from build123d import *

# Parameters (mm, degrees)
SKETCH1_R           = 7.5
BOSS_EXTRUDE2_DEPTH = 2.5
SKETCH1_6_R         = 2.5
CUT_EXTRUDE1_DEPTH  = 3.5
SKETCH1_7_R         = 3.5
SKETCH1_7_R_2       = 2.5
BOSS_EXTRUDE3_DEPTH = 4


with BuildPart() as part:
    # Sketch1 → Boss-Extrude2 (new body)
    with BuildSketch(Plane(origin=(0, 0, 0), x_dir=(1, 0, 0), z_dir=(0, 1, 0))):
        Circle(SKETCH1_R)
    extrude(amount=BOSS_EXTRUDE2_DEPTH)

    # Sketch1<6> → Cut-Extrude1 (cut)
    with BuildSketch(Plane(origin=(0, 0, 0), x_dir=(1, 0, 0), z_dir=(0, 1, 0))):
        Circle(SKETCH1_6_R)
    extrude(amount=CUT_EXTRUDE1_DEPTH, mode=Mode.SUBTRACT)

    # Sketch1<7> → Boss-Extrude3 (add)
    with BuildSketch(Plane(origin=(0, 0, 0), x_dir=(1, 0, 0), z_dir=(0, 1, 0))):
        Circle(SKETCH1_7_R)
        Circle(SKETCH1_7_R_2, mode=Mode.SUBTRACT)
    extrude(amount=BOSS_EXTRUDE3_DEPTH)


solid = part.part
Input: part model. Units: mm. Frame: model coordinates. A direction names the side the tool comes from. Round coordinates to 2 decimals unless told otherwise and drop trailing zeros. Order: outer loops, then holes, each group sorted by start corner. A loop starts at its lowest first (then second) coordinate and runs counter-clockwise, first axis right, second up.
1. Cut plane B-B, the plane z = 2.25. Output: boundary loops of the cut face in (x, y), then the cut area to 3 significant figures.
The answers:
outline: (-7.15, 0) - (-1.09, 0) - (-1.09, 4) - (-2.68, 4) - (-2.68, 2.5) - (-7.15, 2.5) - close; (1.09, 0) - (7.15, 0) - (7.15, 2.5) - (2.68, 2.5) - (2.68, 4) - (1.09, 4) - close
area: 35.1 mm2
2. Cut plane D-D, the plane z = -3. Output: boundary loops of the cut face in (x, y).
The answers:
outline: (-6.87, 0) - (6.87, 0) - (6.87, 2.5) - (1.8, 2.5) - (1.8, 4) - (-1.8, 4) - (-1.8, 2.5) - (-6.87, 2.5) - close
3. Mould query, pull axis Z, two halves, no side actions, for faces 3 (the face through (-2, 0, -2)), 4 (the face through (3.233, 3.24, 1.341)), 5 (the face through (-0.54, 1.97, 2.44)). Classes: released by +Z, released by -Z, zero draft, split by the parting line, or undercut.
The answers:
face 3: zero draft
face 4: split by the parting line
face 5: undercut
4. Set-up query: faces 1 (the face through (2, 4, 2)), 2 (the face through (3.2, 2.5, -1.8)). Return all of +Z, -Z, +X, -X, +Y, -Y with unobstructed straight access to the full face (end or side cutting, diameter ignored); none if empty.
The answers:
face 1: +Z, -Z, +X, -X, +Y
face 2: +Y
5. Cut plane A-A, the plane x = 0. Output: boundary loops of the cut face in (y, z), then the cut area to 3 significant figures.
The answers:
outline: (0, -7.5) - (2.5, -7.5) - (2.5, -3.5) - (4, -3.5) - (4, -2.5) - (0, -2.5) - close; (0, 2.5) - (4, 2.5) - (4, 3.5) - (2.5, 3.5) - (2.5, 7.5) - (0, 7.5) - close
area: 28.0 mm2
6. Material intervals for line 1 (Z direction, x = 0, y = 0.85); line 2 (Z direction, x = 0, y = 2.9), sorted ascending.
The answers:
line 1: z = -7.5 to -2.5, 2.5 to 7.5
line 2: z = -3.5 to -2.5, 2.5 to 3.5
7. Cut plane C-C, the plane y = 2.8. Output: boundary loops of the cut face in (x, z), then the cut area to 3 significant figures.
The answers:
outline: circle Ø7 at (0, 0); hole circle Ø5 at (0, 0)
area: 18.8 mm2
8. Pin query (flat end, axial travel): P1, Ø4.5, axis at x = 0, z = 0, coming from the -Y side; P2, Ø2, axis at y = 2, z = 3.5, coming from the +X side; P3, Ø1, axis at x = 2, y = 0.5, coming from the +Z side. Return the tip coordinate at first contact, or that it passes through.
The answers:
P1: passes through
P2: stops at x = 7.07
P3: stops at z = 7.35
